Autodesk Inventor part; units mm, degrees
ref_plane "YZ Plane" through (0, 0, 0) normal (1, 0, 0) x (0, 1, 0)
ref_plane "XZ Plane" through (0, 0, 0) normal (0, 1, 0) x (-1, 0, 0)
ref_plane "XY Plane" through (0, 0, 0) normal (0, 0, 1) x (1, 0, 0)
sketch "Sketch1" plane through (0, 0, 0) normal (0, 1, 0) x (-1, 0, 0)
  line L0 (0, 0) -> (12, 0)
  line L1 (12, 0) -> (12, -119.5)
  line L2 (12, -119.5) -> (0, -119.5)
  line L3 (0, -119.5) -> (0, 0)
  circle A0 centre (6, -3.7) radius 1.4
  line L4 (6, -113.3) -> (6, -113.3)
  line L5 (4.6, -114.7) -> (4.6, -116.9)
  line L6 (6, -118.3) -> (6, -118.3)
  line L7 (7.4, -116.9) -> (7.4, -114.7)
  arc A1 (7.4, -114.7) -> (6, -113.3) centre (6, -114.7) ccw
  arc A2 (6, -118.3) -> (7.4, -116.9) centre (6, -116.9) ccw
  arc A3 (6, -113.3) -> (4.6, -114.7) centre (6, -114.7) ccw
  arc A4 (4.6, -116.9) -> (6, -118.3) centre (6, -116.9) ccw
  point P0 (4.6, -118.3)
  point P1 (4.6, -113.3)
  dimension "d0" = 12
  dimension "d1" = 119.5
  dimension "d2" = 2.8
  dimension "d3" = 5
  dimension "d4" = 1.4
  dimension "d5" = 2.8
  dimension "d6" = 3.7
  dimension "d7" = 6
  dimension "d8" = 1.2
  dimension "d9" = 6
extrude "Extrusion1" add sketch "Sketch1" along normal blind 4
sketch "Sketch2" plane through (-12, 0, 0) normal (0, 0, 1) x (1, 0, 0)
  line L0 (12, 4) -> (0, 4)
  line L1 (1, 4) -> (11, 4)
  line L2 (11, 4) -> (11, 1)
  line L3 (11, 1) -> (1, 1)
  line L4 (1, 1) -> (1, 4)
  line L5 (0, 0) -> (0, 4)
  line L6 (12, 0) -> (12, 4)
  line L7 (0, 0) -> (12, 0)
  dimension "d12" = 1
  dimension "d13" = 1
  dimension "d14" = 1
extrude "Extrusion2" cut sketch "Sketch2" against normal through all contours L2 L3 L4 L0
sketch "Sketch3" plane through (0, 4, 0) normal (0, 1, 0) x (1, 0, 0)
  line L0 (-12, 119.5) -> (-12, 0)
  line L1 (-11, 0) -> (-11, 119.5)
  line L2 (-12, 17) -> (-11, 17)
  line L3 (-11, 17) -> (-11, 20)
  line L4 (-11, 20) -> (-12, 20)
  line L5 (-12, 20) -> (-12, 17)
  line L6 (-12, 30.5) -> (-11, 30.5)
  line L7 (-11, 30.5) -> (-11, 33.5)
  line L8 (-11, 33.5) -> (-12, 33.5)
  line L9 (-12, 33.5) -> (-12, 30.5)
  line L10 (-12, 86) -> (-11, 86)
  line L11 (-11, 86) -> (-11, 89)
  line L12 (-11, 89) -> (-12, 89)
  line L13 (-12, 89) -> (-12, 86)
  line L14 (-12, 99.5) -> (-11, 99.5)
  line L15 (-11, 99.5) -> (-11, 102.5)
  line L16 (-11, 102.5) -> (-12, 102.5)
  line L17 (-12, 102.5) -> (-12, 99.5)
  line L18 (-1, 0) -> (-1, 119.5)
  line L19 (0, 0) -> (0, 119.5)
  line L20 (0, 99.5) -> (0, 102.5)
  line L21 (-1, 102.5) -> (-1, 99.5)
  line L22 (-1, 88.5) -> (0, 88.5)
  line L23 (0, 88.5) -> (0, 91.5)
  line L24 (0, 91.5) -> (-1, 91.5)
  line L25 (-1, 91.5) -> (-1, 88.5)
  line L26 (-12, 0) -> (-11, 0)
  line L27 (-11, 119.5) -> (-12, 119.5)
  line L28 (0, 119.5) -> (-1, 119.5)
  line L29 (-1, 104.5) -> (0, 104.5)
  line L30 (0, 104.5) -> (0, 101.5)
  line L31 (0, 101.5) -> (-1, 101.5)
  line L32 (-1, 101.5) -> (-1, 104.5)
  point P0 (0, 88.5)
  dimension "d17" = 3
  dimension "d18" = 17
  dimension "d19" = 3
  dimension "d20" = 3
  dimension "d21" = 3
  dimension "d22" = 3
  dimension "d24" = 10.5
  dimension "d25" = 17
  dimension "d26" = 10.5
  dimension "d28" = 1
  dimension "d29" = 3
  dimension "d30" = 15
  dimension "d31" = 10
extrude "Extrusion3" add sketch "Sketch3" along normal blind 1 contours L16 L1 L14 L0 | L12 L1 L10 L0 | L8 L1 L6 L0 | L4 L1 L2 L0 | L18 L24 L19 L22 | L18 L29 L19 L31
sketch "Sketch4" plane through (0, 4, 0) normal (0, 1, 0) x (1, 0, 0)
  line L0 (0, 119.5) -> (-12, 119.5)
  line L1 (-6, 119.5) -> (-6, 59.75) construction
  line L2 (-1, 0) -> (-11, 0)
  circle A0 centre (-6, 3.7) radius 1.4
  circle A1 centre (-6, 59.75) radius 56.05 construction
  point P0 (0, 0)
  dimension "d34" = 59.75
equation "\"d19\" = d17"
equation "\"d20\" = d17"
equation "\"d21\" = d17"
equation "\"d22\" = d17"
properties part number "Barra fijación calefactor" material "Aluminum 6061"
The model under review builds one solid part; all positions refer to its coordinate system, in mm. A direction names the side the tool comes from. Round coordinates to 2 decimals unless told otherwise and drop trailing zeros. Order: outer loops, then holes, each group sorted by start corner. A loop starts at its lowest first (then second) coordinate and runs counter-clockwise, first axis right, second up. Notation, with made-up numbers: (-25, 24) -> (16, 24) arc R19 ccw to (16, 34) -> close; hole circle Ø3 at (53, 52). An arc over 180 degrees is marked (long way). Use CSV: the item, a comma, the result in double quotes. Start each with the question number.
(1) Consider section C-C on y = 2.95. Write out the cut boundary in (x, z).
(2) Wall thickness on probe 1 along Z at (x, y) = (-6, 0.75); probe 2 along X at (y, z) = (1.85, -5.5); probe 3 along X at (y, z) = (0.25, -3.7): over which ranges is each line inside the solid? List them lowest first. Write a range as from..to.
(3) Consider section D-D on z = -74.5. Write out the cut boundary in (x, y), and give its area (3 significant figures).
(4) Mouldability with a two-part tool opening along X and no side actions: class faces 3 (the face through (-6.1, 0.6, -119.5)), 4 (the face through (-1, 3, -59)), 5 (the face through (-12, 2, -59)) as pulls with the +X half, pulls with the -X half, needs draft (parallel to the pull), parting line crosses it, or undercut.
(5) Consider section B-B on x = -6. Write out the cut boundary in (y, z), and give its area (3 significant figures).
(6) Tool access review of faces 1 (the face through (-11, 3, -59)), 2 (the face through (0, 2, -61)): name each direction out of +Z, -Z, +X, -X, +Y, -Y from which nothing blocks a thin tool from reaching the whole face with its end or side.
(7) Insertion check: pin 1 (3 mm diameter, centred on x = -4.5, z = -89, fed in from +Y); pin 2 (0.5 mm diameter, centred on x = -11.5, z = -7, fed in from +Y); pin 3 (0.8 mm diameter, centred on x = -11.5, y = 4.5, fed in from -Z). Each pin has a flat end and moves straight along its axis. Give the tip position at first contact, or say it passes through.
(8) Consider section A-A on z = -3.7. Write out the cut boundary in (x, y), and give its area (3 significant figures).
Responses:
1,outline,"(-12, -119.5) -> (-11, -119.5) -> (-11, 0) -> (-12, 0) -> close; (-1, -119.5) -> (0, -119.5) -> (0, 0) -> (-1, 0) -> close"
2,probe 1,"-119.5..-118.3, -113.3..-5.1, -2.3..0"
2,probe 2,"-12..-11, -1..0"
2,probe 3,"-12..-7.4, -4.6..0"
3,outline,"(-12, 0) -> (0, 0) -> (0, 4) -> (-1, 4) -> (-1, 1) -> (-11, 1) -> (-11, 4) -> (-12, 4) -> close"
3,area,"18.0 mm²"
4,face 3,"needs draft"
4,face 4,"undercut"
4,face 5,"pulls with the -X half"
5,outline,"(0, -119.5) -> (1, -119.5) -> (1, -118.3) -> (0, -118.3) -> close; (0, -113.3) -> (1, -113.3) -> (1, -5.1) -> (0, -5.1) -> close; (0, -2.3) -> (1, -2.3) -> (1, 0) -> (0, 0) -> close"
5,area,"112 mm²"
6,face 1,"+Z, -Z, +Y"
6,face 2,"+Z, -Z, +X, +Y, -Y"
7,pin 1,"y = 1"
7,pin 2,"y = 4"
7,pin 3,"z = -102.5"
8,outline,"(-12, 0) -> (-7.4, 0) -> (-7.4, 1) -> (-11, 1) -> (-11, 4) -> (-12, 4) -> close; (-4.6, 0) -> (0, 0) -> (0, 4) -> (-1, 4) -> (-1, 1) -> (-4.6, 1) -> close"
8,area,"15.2 mm²"
